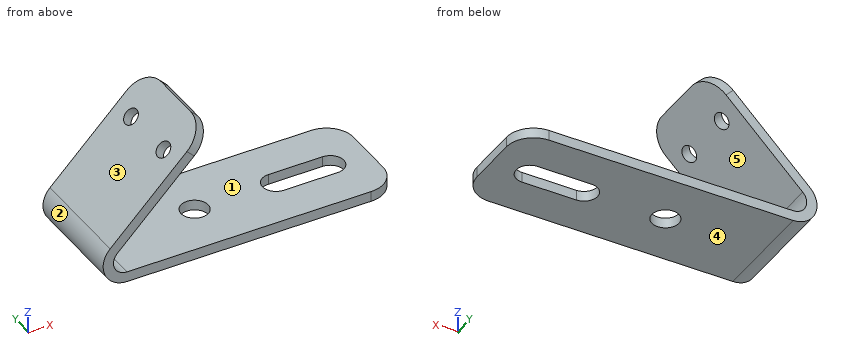
```python
from build123d import *

# Parameters (mm, degrees)
F1_DEPTH = 9.75
F2_R     = 2.5
F3_DEPTH = 2
F4_R     = 1.5
F5_DEPTH = 2
F6_R     = 5


with BuildPart() as f1:
    # F0 (on Front) → F1 (new body, symmetric)
    with BuildSketch(Plane.XZ):
        with BuildLine():
            Line((14.5664, 20.788939), (-3.11127, 3.11127))
            ThreePointArc((-3.11127, 3.11127), (-4.06507, -1.683807), (0, -4.4))
            Line((0, -4.4), (50, -4.4))
            Line((50, -4.4), (50, -2.5))
            Line((50, -2.5), (0, -2.5))
            ThreePointArc((0, -2.5), (-2.309699, -0.956709), (-1.767767, 1.767767))
            Line((-1.767767, 1.767767), (15.909903, 19.445436))
            Line((15.909903, 19.445436), (14.5664, 20.788939))
        make_face()
    extrude(amount=F1_DEPTH, both=True)

    # F2 (on face) → F3 (cut)
    with BuildSketch(Plane(origin=(0, 0, -4.4), x_dir=(1, 0, 0), z_dir=(0, 0, -1))):
        with Locations((18, 0)):
            Circle(F2_R)
        with BuildLine():
            Line((43, 2.5), (33, 2.5))
            ThreePointArc((33, 2.5), (30.5, 0), (33, -2.5))
            Line((33, -2.5), (43, -2.5))
            ThreePointArc((43, -2.5), (45.5, 0), (43, 2.5))
        make_face()
    extrude(amount=-F3_DEPTH, mode=Mode.SUBTRACT)

    # F4 (on face) → F5 (cut)
    with BuildSketch(Plane(origin=(-3.11127, 0, 3.11127), x_dir=(0, -1, 0), z_dir=(-0.707107, 0, 0.707107))):
        with Locations((-5.25, 17.5)):
            Circle(F4_R)
        with Locations((5.25, 17.5)):
            Circle(F4_R)
    extrude(amount=-F5_DEPTH, mode=Mode.SUBTRACT)

    # F6
    f6_edges = [f1.edges().sort_by_distance(p)[0] for p in [
        (15.238151, -9.75, 20.117188),
        (15.238151, 9.75, 20.117188),
        (50, 9.75, -3.45),
        (50, -9.75, -3.45),
    ]]
    fillet(f6_edges, radius=F6_R)


solid = f1.part
```
Can you work these out from the model? Positions are in its coordinate system, mm. Face numbers are marked on the shaded views. A direction names the side the tool comes from. Coordinates: 2 decimals unless noted, no trailing zeros. Loops run counter-clockwise (first coordinate to the right, second up) from the corner with the lowest first, then second, coordinate; pieces in that order, holes last.
Item 1: Please list where these lines run through material, in increasing order: L1, parallel to Y at x = 18, z = -3.75; L2, parallel to X at y = 0, z = -3.45; L3, parallel to X at y = 0, z = -3.6.
Answers below:
L1: y = -9.75 to -2.5, 2.5 to 9.75
L2: x = -2.73 to 15.5, 20.5 to 30.5, 45.5 to 50
L3: x = -2.53 to 15.5, 20.5 to 30.5, 45.5 to 50
Item 2: Suppose I cut it at A-A (y = 0). Please give me the cut outline in (x, z).
Answers below:
outline: (-3.11, 3.11) arc R4.4 ccw to (0, -4.4) - (15.5, -4.4) - (15.5, -2.5) - (0, -2.5) arc R2.5 cw to (-1.77, 1.77) - (15.91, 19.45) - (14.57, 20.79) - close; (20.5, -4.4) - (30.5, -4.4) - (30.5, -2.5) - (20.5, -2.5) - close; (45.5, -4.4) - (50, -4.4) - (50, -2.5) - (45.5, -2.5) - close
Item 3: Suppose I cut it at B-B (x = 18). Please give me the cut outline in (y, z), then the cut area to 4 significant figures.
Answers below:
outline: (-9.75, -4.4) - (-2.5, -4.4) - (-2.5, -2.5) - (-9.75, -2.5) - close; (2.5, -4.4) - (9.75, -4.4) - (9.75, -2.5) - (2.5, -2.5) - close
area: 27.55 mm2
Item 4: Suppose I cut it at D-D (z = 1). Please give me the cut outline in (x, y).
Answers below:
outline: (-4.28, -9.75) - (-2.29, -9.75) - (-2.29, 9.75) - (-4.28, 9.75) - close
Item 5: If we mould it in two halves opening along Z, with no side actions, what happens to the marked faces 3, 4 and 5? For each: released by +Z, released by -Z, zero draft, split by the parting line, or undercut.
Answers below:
face 3: released by +Z
face 4: released by -Z
face 5: undercut
Item 6: Which directions (+Z, -Z, +X, -X, +Y, -Y) give clear straight access to the entire face, cutting with the end or side of a thin tool? Please do the marked faces 1 and 2.
Answers below:
face 1: +X, +Y, -Y
face 2: -X, +Y, -Y
Item 7: I'm going to push flat-ended pins straight in: pin 1 (1 mm diameter, centred on x = 31.5, y = 5.5, fed in from +Z); pin 2 (4.5 mm diameter, centred on x = 18, y = 0, fed in from +Z); pin 3 (4 mm diameter, centred on y = 5.5, z = 10.5, fed in from +X). Where does each tip first touch, or does it pass through?
Answers below:
pin 1: stops at z = -2.5
pin 2: stops at z = 19.61
pin 3: stops at x = 8.96
Item 8: Suppose I cut it at C-C (y = 8.5). Please give me the cut outline in (x, z), then the cut area to 3 significant figures.
Answers below:
outline: (-3.11, 3.11) arc R4.4 ccw to (0, -4.4) - (48.31, -4.4) - (48.31, -2.5) - (0, -2.5) arc R2.5 cw to (-1.77, 1.77) - (14.71, 18.25) - (13.37, 19.59) - close
area: 152 mm2
